Geometry: final body of the model. Coordinates: model frame, mm. A direction names the side the tool comes from. Round coordinates to 2 decimals unless told otherwise and drop trailing zeros. Write each loop counter-clockwise with the first axis right and the second up, starting at its lowest first coordinate (ties: lowest second). Pieces come first, ordered by that corner, then holes.
from build123d import *

# Parameters (mm, degrees)
TABAN_FLAN_1_DEPTH = 64


# Sheet-metal steps are written as plain solids
with BuildPart() as part:
    # Çizim1 → Taban-Flanş1 (new body)
    with BuildSketch(Plane.YZ):
        with BuildLine():
            Line((0, 0), (0, 23.5))
            ThreePointArc((0, 23.5), (2.5, 26), (5, 23.5))
            Line((5, 23.5), (5, 0))
            Line((5, 0), (6, 0))
            Line((6, 0), (6, 23.5))
            ThreePointArc((6, 23.5), (2.5, 27), (-1, 23.5))
            Line((-1, 23.5), (-1, 0))
            Line((-1, 0), (0, 0))
        make_face()
    extrude(amount=TABAN_FLAN_1_DEPTH)


solid = part.part
1) Section C-C on y = 2.5. Output: boundary loops of the cut face in (x, z).
2) Section B-B on x = 31.5. Output: boundary loops of the cut face in (y, z).
3) Section A-A on z = 11.25. Output: boundary loops of the cut face in (x, y), plus the area to 3 significant figures.
4) Line query: probe 1 along Y at (x, z) = (47, 23.5); probe 2 along Y at (x, z) = (37, 24); probe 3 along Z at (x, y) = (45, 1.25). Output: solid intervals per line, ascending.
5) First-contact query: P1, Ø1.5, axis at x = 52, y = 3.5, coming from the +Z side. Flat tip, straight axial feed; report the tip coordinate or a pass-through.
6) Reachability of faces 1 (the flat face through (32, 6, 12)), 2 (the flat face through (32, 0, 12)) from +Z, -Z, +X, -X, +Y, -Y: full face, straight path, thin tool, end or side. Return the list, or none.
Filled in:
1. outline: (0, 26) - (64, 26) - (64, 27) - (0, 27) - close
2. outline: (-1, 0) - (0, 0) - (0, 23.5) arc R2.5 cw to (5, 23.5) - (5, 0) - (6, 0) - (6, 23.5) arc R3.5 ccw to (-1, 23.5) - close
3. outline: (0, -1) - (64, -1) - (64, 0) - (0, 0) - close; (0, 5) - (64, 5) - (64, 6) - (0, 6) - close
3. area: 128 mm2
4. probe 1: y = -1 to 0, 5 to 6
4. probe 2: y = -0.96 to 0.05, 4.95 to 5.96
4. probe 3: z = 25.67 to 26.77
5. P1: stops at z = 26.99
6. face 1: +Z, -Z, +X, -X, +Y
6. face 2: -Z, +X, -X
